from build123d import *

# Parameters (mm, degrees)
F1_DEPTH = 9.525
F2_R     = 0.635
F3_R     = 1.27


with BuildPart() as f1:
    # F0 (on Front) → F1 (new body, symmetric)
    with BuildSketch(Plane.XZ):
        with BuildLine():
            Line((0, 0.762), (0, 0))
            Line((0, 0), (6.35, 0))
            Line((6.35, 0), (1.27, 8.798818))
            ThreePointArc((1.27, 8.798818), (1.774167, 10.55545), (3.51186, 9.989443))
            Line((3.51186, 9.989443), (11.29061, -5.99866))
            Line((11.29061, -5.99866), (11.975814, -5.665285))
            Line((11.975814, -5.665285), (4.197064, 10.322818))
            ThreePointArc((4.197064, 10.322818), (1.416755, 11.22843), (0.610089, 8.417818))
            Line((0.610089, 8.417818), (5.030177, 0.762))
            Line((5.030177, 0.762), (0, 0.762))
        make_face()
        with BuildLine():
            Line((-6.35, 0), (0, 0))
            Line((0, 0), (0, 0.762))
            Line((0, 0.762), (-5.030177, 0.762))
            Line((-5.030177, 0.762), (-0.610089, 8.417818))
            ThreePointArc((-0.610089, 8.417818), (-1.416755, 11.22843), (-4.197064, 10.322818))
            Line((-4.197064, 10.322818), (-11.975814, -5.665285))
            Line((-11.975814, -5.665285), (-11.29061, -5.99866))
            Line((-11.29061, -5.99866), (-3.51186, 9.989443))
            ThreePointArc((-3.51186, 9.989443), (-1.774167, 10.55545), (-1.27, 8.798818))
            Line((-1.27, 8.798818), (-6.35, 0))
        make_face()
    extrude(amount=F1_DEPTH, both=True)

    # F2
    f2_edges = [f1.edges().sort_by_distance(p)[0] for p in [
        (6.35, 0, 0),
        (-6.35, 0, 0),
    ]]
    fillet(f2_edges, radius=F2_R)

    # F3
    f3_edges = [f1.edges().sort_by_distance(p)[0] for p in [
        (5.030177, 0, 0.762),
        (-5.030177, 0, 0.762),
    ]]
    fillet(f3_edges, radius=F3_R)


solid = f1.part
Could you check a few things on this model? Use its own coordinates, in mm. A direction names the side the tool comes from. Give positions to 0.01 mm unless a question says otherwise; leave off trailing zeros. Order: outer loops, then holes, each group sorted by start corner. A loop starts at its lowest first (then second) coordinate and runs counter-clockwise, first axis right, second up.
1. For faces 5 (the flat face through (-8.032, -0.133, 2.441)), 6 (the flat face through (2.25, -0.13, 5.58)), which set-ups out of +Z, -Z, +X, -X, +Y, -Y let a thin tool reach every point of the face, with its end or its side?
2. I need wall thicknesses on L1, parallel to X at y = -8.25, z = 4.75; L2, parallel to X at y = -0.25, z = 10; L3, parallel to Z at x = -2, y = -3.25. Which ranges of each line are inside material? Lowest first, please.
3. Suppose I cut it at B-B (x = -4.5). List the corners of the cut face in (y, z) for me (3 decimals).
4. Suppose I cut it at C-C (y = 2.5). List the corners of the cut face in (x, z) for me (1 decimal).
5. Will these pins go through, and if not, where does the flat tip stop? P1, Ø1.5, axis at x = 9, z = 5, coming from the -Y side; P2, Ø1, axis at x = -6.5, y = 7.5, coming from the +Z side; P3, Ø6, axis at x = 6, y = 1.5, coming from the +Z side; P4, Ø3, axis at x = -3, y = -7.5, coming from the -Z side.
6. We'd pull the mould along Z, two halves only. Please class faces 1 (the cylindrical face through (-3.92, -0.13, 1.38)), 2 (the flat face through (-3, 9.525, 5)), 3 (the flat face through (0, 0, 0)), 4 (the flat face through (8.14, -0.13, 2.22)): pulls with the +Z half, pulls with the -Z half, needs draft (parallel to the pull), parting line crosses it, or undercut.
7. Suppose I cut it at D-D (z = 9.5). List the corners of the cut face in (x, y) for me (3 decimals), plus the area to 3 significant figures.
8. Suppose I cut it at A-A (x = -2). List the corners of the cut face in (y, z) for me (3 decimals).
Solved:
1. face 5: +Z, -X, +Y, -Y
1. face 6: +Y, -Y
2. L1: x = -6.91 to -6.06, -3.61 to -2.73, 2.73 to 3.61, 6.06 to 6.91
2. L2: x = -4.35 to -3.51, -1.23 to -0.42, 0.42 to 1.23, 3.51 to 4.35
2. L3: z = 0 to 0.76, 6.01 to 7.53, 10.65 to 11.43
3. outline: (-9.525, 0) - (9.525, 0) - (9.525, 3.204) - (-9.525, 3.204) - close; (-9.525, 7.958) - (9.525, 7.958) - (9.525, 9.7) - (-9.525, 9.7) - close
4. outline: (-12, -5.7) - (-11.3, -6) - (-3.5, 10) arc R1.3 cw (long way) to (-1.3, 8.8) - (-5.8, 1) arc R0.6 ccw to (-5.3, 0) - (5.3, 0) arc R0.6 ccw to (5.8, 1) - (1.3, 8.8) arc R1.3 cw (long way) to (3.5, 10) - (11.3, -6) - (12, -5.7) - (4.2, 10.3) arc R2 ccw (long way) to (0.6, 8.4) - (3.9, 2.7) arc R1.3 cw to (2.8, 0.8) - (-2.8, 0.8) arc R1.3 cw to (-3.9, 2.7) - (-0.6, 8.4) arc R2 ccw (long way) to (-4.2, 10.3) - close
5. P1: passes through
5. P2: stops at z = 6.62
5. P3: stops at z = 11.37
5. P4: stops at z = 0
6. face 1: undercut
6. face 2: needs draft
6. face 3: pulls with the -Z half
6. face 4: pulls with the +Z half
7. outline: (-4.597, -9.525) - (-3.75, -9.525) - (-3.75, 9.525) - (-4.597, 9.525) - close; (-1.102, -9.525) - (-0.339, -9.525) - (-0.339, 9.525) - (-1.102, 9.525) - close; (0.339, -9.525) - (1.102, -9.525) - (1.102, 9.525) - (0.339, 9.525) - close; (3.75, -9.525) - (4.597, -9.525) - (4.597, 9.525) - (3.75, 9.525) - close
7. area: 61.3 mm2
8. outline: (-9.525, 0) - (9.525, 0) - (9.525, 0.762) - (-9.525, 0.762) - close; (-9.525, 6.01) - (9.525, 6.01) - (9.525, 7.534) - (-9.525, 7.534) - close; (-9.525, 10.649) - (9.525, 10.649) - (9.525, 11.432) - (-9.525, 11.432) - close
